```python
from build123d import *

# Parameters (mm, degrees)
F0_W     = 22
F0_H     = 28
F1_DEPTH = 3.5
F2_R     = 4.25
F2_R_2   = 1.75
F3_DEPTH = 2
F4_DEPTH = 3.501
F5_W     = 22
F5_H     = 6
F5_R     = 1.75
F6_DEPTH = 1.5
F7_DEPTH = 4.5


with BuildPart() as f1:
    # F0 (on Top) → F1 (new body)
    with BuildSketch(Plane.XY):
        with Locations((1.8137441948, -6.2994613256)):
            Rectangle(F0_W, F0_H)
    extrude(amount=F1_DEPTH)

    # F2 (on face) → F3 (cut)
    with BuildSketch(Plane.XY.offset(3.5)):
        with Locations((1.8137441948, 0.4505386744)):
            Circle(F2_R)
        with Locations((1.8137441948, 0.4505386744)):
            Circle(F2_R_2, mode=Mode.SUBTRACT)
    extrude(amount=-F3_DEPTH, mode=Mode.SUBTRACT)

    # F4 (cut, through all): a face of the model
    f4_faces = [f1.faces().sort_by_distance(p)[0] for p in [
        (1.8137441948, 0.4505386744, 3.5),
    ]]
    extrude(f4_faces, amount=-F4_DEPTH, mode=Mode.SUBTRACT)

    # F5 (on face) → F6 (join)
    with BuildSketch(Plane(origin=(0, 0, 0), x_dir=(1, 0, 0), z_dir=(0, 0, -1))):
        with Locations((1.8137441948, -0.4505386744)):
            Rectangle(F5_W, F5_H)
        with Locations((1.8137441948, -0.4505386744)):
            Circle(F5_R, mode=Mode.SUBTRACT)
    extrude(amount=F6_DEPTH)

    # F2 (on face) → F7 (join)
    with BuildSketch(Plane.XY.offset(3.5)):
        with BuildLine():
            ThreePointArc((-9.1862558052, -11.2994613256), (1.4435215802, -5.8944727122), (12.8137441948, -2.2994613256))
            Line((12.8137441948, -2.2994613256), (12.8137441948, 7.7005386744))
            Line((12.8137441948, 7.7005386744), (-9.1862558052, 7.7005386744))
            Line((-9.1862558052, 7.7005386744), (-9.1862558052, -11.2994613256))
        make_face()
        with Locations((1.8137441948, 0.4505386744)):
            Circle(F2_R, mode=Mode.SUBTRACT)
    extrude(amount=F7_DEPTH)


solid = f1.part
```
The model under review builds one solid part; all positions refer to its coordinate system, in mm. A direction names the side the tool comes from. Coordinates: 2 decimals unless noted, no trailing zeros. Write each loop counter-clockwise with the first axis right and the second up, starting at its lowest first coordinate (ties: lowest second). Pieces come first, ordered by that corner, then holes.
1) Machinability: for faces 4 (the face through (2, -13, 3.5)), 5 (the face through (2, -2.549, -1)), 6 (the face through (4, 1, 1.5)), which of the approach directions +Z, -Z, +X, -X, +Y, -Y give a long, thin tool a straight path to every point of the face, cutting with its end or side? Answer none if there is none.
2) We need section A-A on y = -0.25. State the section outline as (x, z) points.
3) Clearance check with flat-ended pins moving along their axes: pin 1 Ø0.8 at (x, z) = (-0.5, -1) entering from +Y; pin 2 Ø7.5 at (x, y) = (1.81, 0.45) entering from +Z; pin 3 Ø9 at (x, y) = (7, -14) entering from -Z. State where each tip first meets the part, or that it passes through.
4) We need section D-D on z = 5.25. State the section outline as (x, y) points.
5) To check wall thickness, follow probe 1 along Z at (x, y) = (4.25, -10); probe 2 along Y at (x, z) = (1, 2.25); probe 3 along Y at (x, z) = (1, 7.25). State the ranges of each line that lie inside material, in increasing order.
6) The part is to be moulded in two halves that separate along Y. For faces 1 (the face through (2, 3.451, -1)), 2 (the face through (2.75, -1.03, 0.02)), 3 (the face through (2, 6, 0)), say which applies: pulls with the +Y half, pulls with the -Y half, needs draft (parallel to the pull), parting line crosses it, or undercut.
7) We need section B-B on x = 0.5. State the section outline as (y, z) points, then the cut area to 3 significant figures.
8) We need section C-C on x = 10.75. State the section outline as (y, z) points.
Answer list:
1. face 4: +Z, +X, -Y
1. face 5: -Z, +X, -X, -Y
1. face 6: +Z
2. outline: (-9.19, -1.5) - (0.21, -1.5) - (0.21, 1.5) - (-2.38, 1.5) - (-2.38, 8) - (-9.19, 8) - close; (3.42, -1.5) - (12.81, -1.5) - (12.81, 8) - (6.01, 8) - (6.01, 1.5) - (3.42, 1.5) - close
3. pin 1: stops at y = 3.45
3. pin 2: stops at z = 1.5
3. pin 3: stops at z = 0
4. outline: (-9.19, -11.3) arc R72.72 cw to (12.81, -2.3) - (12.81, 7.7) - (-9.19, 7.7) - close; hole circle Ø8.5 at (1.81, 0.45)
5. probe 1: z = 0 to 3.5
5. probe 2: y = -20.3 to -3.72, 4.62 to 7.7
5. probe 3: y = -6.08 to -3.72, 4.62 to 7.7
6. face 1: pulls with the +Y half
6. face 2: undercut
6. face 3: needs draft
7. outline: (-20.3, 0) - (-2.55, 0) - (-2.55, -1.5) - (-0.71, -1.5) - (-0.71, 1.5) - (-3.59, 1.5) - (-3.59, 8) - (-6.29, 8) - (-6.29, 3.5) - (-20.3, 3.5) - close; (1.61, -1.5) - (3.45, -1.5) - (3.45, 0) - (7.7, 0) - (7.7, 8) - (4.49, 8) - (4.49, 1.5) - (1.61, 1.5) - close
7. area: 110 mm2
8. outline: (-20.3, 0) - (-2.55, 0) - (-2.55, -1.5) - (3.45, -1.5) - (3.45, 0) - (7.7, 0) - (7.7, 8) - (-2.8, 8) - (-2.8, 3.5) - (-20.3, 3.5) - close
